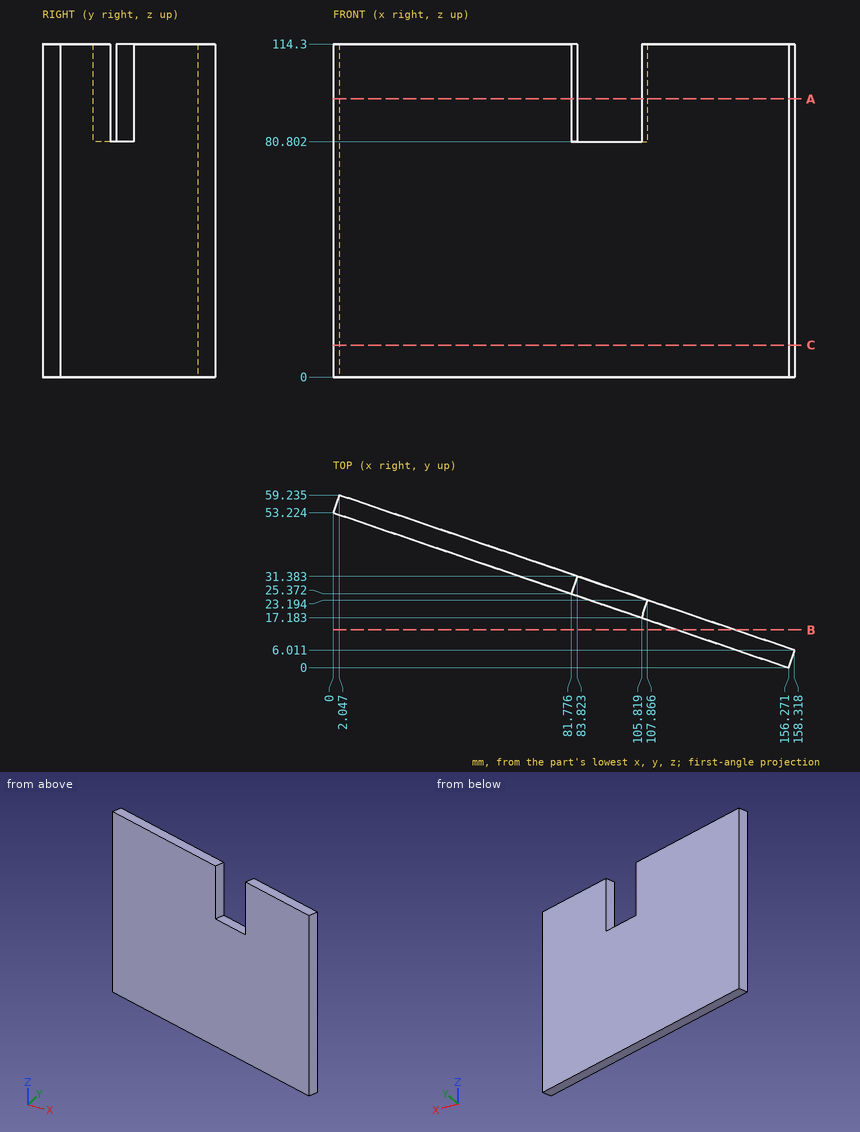
The figure shows three views and two pictorial views of one solid part (mm, origin at its lowest corner). Answer the questions. Coordinates: 2 decimals unless noted, no trailing zeros. Loops run counter-clockwise (first coordinate to the right, second up) from the corner with the lowest first, then second, coordinate; pieces in that order, holes last. Notation, with made-up numbers: (46, 9.25) -> (102, 9.25) arc R20 cw to (102, 26.25) -> close; hole circle Ø6 at (75.25, 81). An arc over 180 degrees is marked (long way). Write item = value, one per line. Start each with the question number.
1) A cutting plane is placed at A-A (z = 95.5). Give the vertices of the cut face in (x, y) (1 decimal).
2) A cutting plane is placed at B-B (y = 13). Give the vertices of the cut face in (x, z), then the cut area to 3 significant figures.
3) A cutting plane is placed at C-C (z = 11). Give the vertices of the cut face in (x, y) (1 decimal).
4) Straight lines are drawn through the part: line 1 (Y direction, x = 52, z = 49.5); line 2 (Y direction, x = 17, z = 41.5) (1 decimal). For each, find the intervals that lie inside material, in ascending order. Write a range as from..to.
5) Given pin 1 Ø4 at (x, z) = (86.5, 47.5) entering from -Y; pin 2 Ø6 at (x, z) = (99.5, 28) entering from -Y; pin 3 Ø3 at (x, z) = (130.5, 86.5) entering from +Y, each flat-ended and moving along its own axis, determine where each tip first touches the part or whether it passes through.
Responses:
q1.outline = (0, 53.2) -> (81.8, 25.4) -> (83.8, 31.4) -> (2, 59.2) -> close; (105.8, 17.2) -> (156.3, 0) -> (158.3, 6) -> (107.9, 23.2) -> close
q2.outline = (118.1, 0) -> (137.8, 0) -> (137.8, 114.3) -> (118.1, 114.3) -> close
q2.area = 2,250 mm²
q3.outline = (0, 53.2) -> (156.3, 0) -> (158.3, 6) -> (2, 59.2) -> close
q4.line_1 = 35.51..42.22
q4.line_2 = 47.4..54.1
q5.pin_1 = 23.08
q5.pin_2 = 18.31
q5.pin_3 = 16
